Model file for the job. Use its own axes, mm. Face numbers are marked on the shaded views. A direction names the side the tool comes from. Give positions to 0.01 mm unless a question says otherwise; leave off trailing zeros. Write each loop counter-clockwise with the first axis right and the second up, starting at its lowest first coordinate (ties: lowest second). Pieces come first, ordered by that corner, then holes.
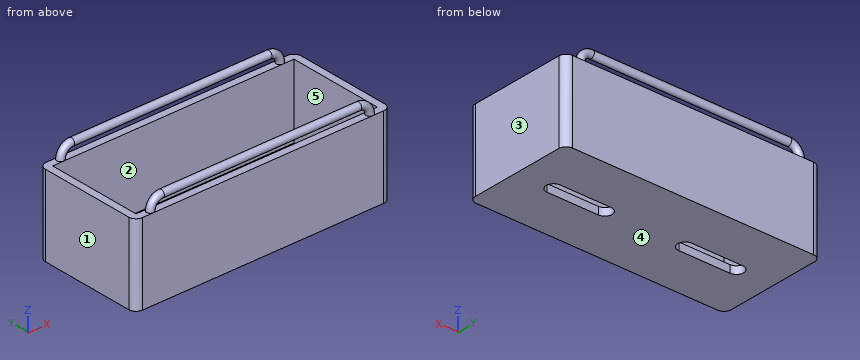
```python
from build123d import *

# Parameters (mm, degrees)
CROQUIS1_W              = 70
CROQUIS1_H              = 30
SALIENTE_EXTRUIR4_DEPTH = 22.045635187
CROQUIS5_W              = 66
CROQUIS5_H              = 26
CORTAR_EXTRUIR1_DEPTH   = 20
CORTAR_EXTRUIR3_DEPTH   = 20
REDONDEO2_R             = 2
REDONDEO3_R             = 2
REDONDEO4_R             = 2
REDONDEO5_R             = 2
BARRER8_OUTLINE_R       = 1
BARRER8_ANGLE           = 90
BARRER8_2_OUTLINE_R     = 1
BARRER8_2_ANGLE         = 90
BARRER8_START           = 21
BARRER8_3_OUTLINE_R     = 1
BARRER8_3_DEPTH         = 1.046635287
BARRER8_START_2         = 7.9899999
BARRER8_4_OUTLINE_R     = 1
BARRER8_4_DEPTH         = 54.0110002
BARRER8_5_OUTLINE_R     = 1
BARRER8_5_DEPTH         = 1.055635287
BARRER9_OUTLINE_R       = 1
BARRER9_ANGLE           = 90
BARRER9_2_OUTLINE_R     = 1
BARRER9_2_ANGLE         = 90
BARRER9_START           = 21
BARRER9_3_OUTLINE_R     = 1
BARRER9_3_DEPTH         = 1.046635287
BARRER9_START_2         = 7.9989999
BARRER9_4_OUTLINE_R     = 1
BARRER9_4_DEPTH         = 54.0020002
BARRER9_5_OUTLINE_R     = 1
BARRER9_5_DEPTH         = 1.046635287


with BuildPart() as part:
    # Croquis1 → Saliente-Extruir4 (new body)
    with BuildSketch(Plane.XY):
        with Locations((35, 15)):
            Rectangle(CROQUIS1_W, CROQUIS1_H)
    extrude(amount=SALIENTE_EXTRUIR4_DEPTH)

    # Croquis5 → Cortar-Extruir1 (cut)
    with BuildSketch(Plane.XY.offset(22.045635187)):
        with Locations((35, 15)):
            Rectangle(CROQUIS5_W, CROQUIS5_H)
    extrude(amount=-CORTAR_EXTRUIR1_DEPTH, mode=Mode.SUBTRACT)

    # Croquis6 → Cortar-Extruir3 (cut)
    with BuildSketch(Plane.XY.offset(2.045635187)):
        with BuildLine():
            Line((10, 17), (24, 17))
            ThreePointArc((24, 17), (26, 15), (24, 13))
            Line((24, 13), (10, 13))
            ThreePointArc((10, 13), (8, 15), (10, 17))
        make_face()
        with BuildLine():
            Line((60, 17), (46, 17))
            ThreePointArc((46, 17), (44, 15), (46, 13))
            Line((46, 13), (60, 13))
            ThreePointArc((60, 13), (62, 15), (60, 17))
        make_face()
    extrude(amount=-CORTAR_EXTRUIR3_DEPTH, mode=Mode.SUBTRACT)

    # Redondeo2
    redondeo2_edges = [part.edges().sort_by_distance(p)[0] for p in [
        (70, 0, 11.022817594),
    ]]
    fillet(redondeo2_edges, radius=REDONDEO2_R)

    # Redondeo3
    redondeo3_edges = [part.edges().sort_by_distance(p)[0] for p in [
        (70, 30, 11.022817594),
    ]]
    fillet(redondeo3_edges, radius=REDONDEO3_R)

    # Redondeo4
    redondeo4_edges = [part.edges().sort_by_distance(p)[0] for p in [
        (0, 0, 11.022817594),
    ]]
    fillet(redondeo4_edges, radius=REDONDEO4_R)

    # Redondeo5
    redondeo5_edges = [part.edges().sort_by_distance(p)[0] for p in [
        (0, 30, 11.022817594),
    ]]
    fillet(redondeo5_edges, radius=REDONDEO5_R)

    # Barrer8 3 outline → Barrer8 3 (add)
    with BuildSketch(Plane.XY.offset(BARRER8_START)):
        with Locations((65, 1)):
            Circle(BARRER8_3_OUTLINE_R)
    extrude(amount=BARRER8_3_DEPTH)



with BuildPart() as body_2:
    # Barrer8: read off the stored shape, not the designer's step
    # Barrer8 outline → Barrer8 (revolve)
    with BuildSketch(Plane(origin=(62.001, 0, 22.046635187), x_dir=(0, 0, 1), z_dir=(-1, 0, 0))):
        with Locations((2.999, 1)):
            Circle(BARRER8_OUTLINE_R)
    revolve(axis=Axis((62.001, 0, 22.046635187), (0, 1, 0)), revolution_arc=BARRER8_ANGLE)



with BuildPart() as body_3:
    # Barrer8 2 outline → Barrer8 2 (revolve)
    with BuildSketch(Plane(origin=(7.99, 0, 22.055635187), x_dir=(-1, 0, 0), z_dir=(0, 0, -1))):
        with Locations((2.99, 1)):
            Circle(BARRER8_2_OUTLINE_R)
    revolve(axis=Axis((7.99, 0, 22.055635187), (0, 1, 0)), revolution_arc=BARRER8_2_ANGLE)


with BuildPart() as body_2_1:
    add(body_2.part)

    add(body_3.part)  # Barrer8 4 merges body 3
    # Barrer8 4 outline → Barrer8 4 (add)
    with BuildSketch(Plane.YZ.offset(BARRER8_START_2)):
        with Locations((1, 25.045635187)):
            Circle(BARRER8_4_OUTLINE_R)
    extrude(amount=BARRER8_4_DEPTH)


with BuildPart() as part_1:
    add(part.part)

    add(body_2_1.part)  # Barrer8 5 merges body 2
    # Barrer8 5 outline → Barrer8 5 (add)
    with BuildSketch(Plane.XY.offset(BARRER8_START)):
        with Locations((5, 1)):
            Circle(BARRER8_5_OUTLINE_R)
    extrude(amount=BARRER8_5_DEPTH)

    # Barrer9 3 outline → Barrer9 3 (add)
    with BuildSketch(Plane.XY.offset(BARRER9_START)):
        with Locations((5, 29)):
            Circle(BARRER9_3_OUTLINE_R)
    extrude(amount=BARRER9_3_DEPTH)



with BuildPart() as body_2_2:
    # Barrer9: read off the stored shape, not the designer's step
    # Barrer9 outline → Barrer9 (revolve)
    with BuildSketch(Plane(origin=(7.999, 0, 22.046635187), x_dir=(-1, 0, 0), z_dir=(0, 0, -1))):
        with Locations((2.999, 29)):
            Circle(BARRER9_OUTLINE_R)
    revolve(axis=Axis((7.999, 0, 22.046635187), (0, 1, 0)), revolution_arc=BARRER9_ANGLE)



with BuildPart() as body_3_2:
    # Barrer9 2 outline → Barrer9 2 (revolve)
    with BuildSketch(Plane(origin=(62.001, 0, 22.046635187), x_dir=(0, 0, 1), z_dir=(-1, 0, 0))):
        with Locations((2.999, 29)):
            Circle(BARRER9_2_OUTLINE_R)
    revolve(axis=Axis((62.001, 0, 22.046635187), (0, 1, 0)), revolution_arc=BARRER9_2_ANGLE)


with BuildPart() as body_2_2_1:
    add(body_2_2.part)

    add(body_3_2.part)  # Barrer9 4 merges body 3 2
    # Barrer9 4 outline → Barrer9 4 (add)
    with BuildSketch(Plane.YZ.offset(BARRER9_START_2)):
        with Locations((29, 25.045635187)):
            Circle(BARRER9_4_OUTLINE_R)
    extrude(amount=BARRER9_4_DEPTH)


with BuildPart() as part_2:
    add(part_1.part)

    add(body_2_2_1.part)  # Barrer9 5 merges body 2 2
    # Barrer9 5 outline → Barrer9 5 (add)
    with BuildSketch(Plane.XY.offset(BARRER9_START)):
        with Locations((65, 29)):
            Circle(BARRER9_5_OUTLINE_R)
    extrude(amount=BARRER9_5_DEPTH)


solid = part_2.part
```
1. Slice it at A-A, the plane z = 19.25. Write the cut outline in (x, y).
Calculated:
outline: (0, 2) arc R2 ccw to (2, 0) - (68, 0) arc R2 ccw to (70, 2) - (70, 28) arc R2 ccw to (68, 30) - (2, 30) arc R2 ccw to (0, 28) - close; hole (2, 2) - (68, 2) - (68, 28) - (2, 28) - close
2. Probe probe 1 along Y at (x, z) = (58, 10.75); probe 2 along X at (y, z) = (5, 7.25); probe 3 along Z at (x, y) = (26.5, 15.5). List the from-to ranges inside material, lowest first.
Calculated:
probe 1: y = 0 to 2, 28 to 30
probe 2: x = 0 to 2, 68 to 70
probe 3: z = 0 to 2.05
3. Slice it at C-C, the plane y = 15. Write the cut outline in (x, z).
Calculated:
outline: (0, 0) - (8, 0) - (8, 2.05) - (2, 2.05) - (2, 22.05) - (0, 22.05) - close; (26, 0) - (44, 0) - (44, 2.05) - (26, 2.05) - close; (62, 0) - (70, 0) - (70, 22.05) - (68, 22.05) - (68, 2.05) - (62, 2.05) - close
4. Pull direction X, two halves, no side cores. Call the marked faces 3, 4 and 5: +X half, -X half, draft (parallel to the pull), parting line (faces both ways), or undercut.
Calculated:
face 3: +X half
face 4: draft
face 5: undercut
5. Slice it at D-D, the plane y = 9.5. Write the cut outline in (x, z), and give its area (3 significant figures).
Calculated:
outline: (0, 0) - (70, 0) - (70, 22.05) - (68, 22.05) - (68, 2.05) - (2, 2.05) - (2, 22.05) - (0, 22.05) - close
area: 223 mm2
6. Which spindle directions (+Z, -Z, +X, -X, +Y, -Y) get a long thin tool onto all of the face, cutting with end or side? Do the marked faces 1 and 2. Say none if no direction does.
Calculated:
face 1: +Z, -Z, -X, +Y, -Y
face 2: +Z
7. Pin check, flat tips, straight feed: P1, Ø6, axis at x = 19, y = 13.5, coming from the +Z side; P2, Ø4, axis at x = 1.5, y = 12.5, coming from the +Z side. Stop position of each tip, or through.
Calculated:
P1: stops at z = 2.05
P2: stops at z = 22.05
8. Slice it at B-B, the plane x = 32. Write the cut outline in (y, z), and give its area (3 significant figures).
Calculated:
outline: (0, 0) - (30, 0) - (30, 22.05) - (28, 22.05) - (28, 2.05) - (2, 2.05) - (2, 22.05) - (0, 22.05) - close; circle Ø2 at (1, 25.05); circle Ø2 at (29, 25.05)
area: 148 mm2
